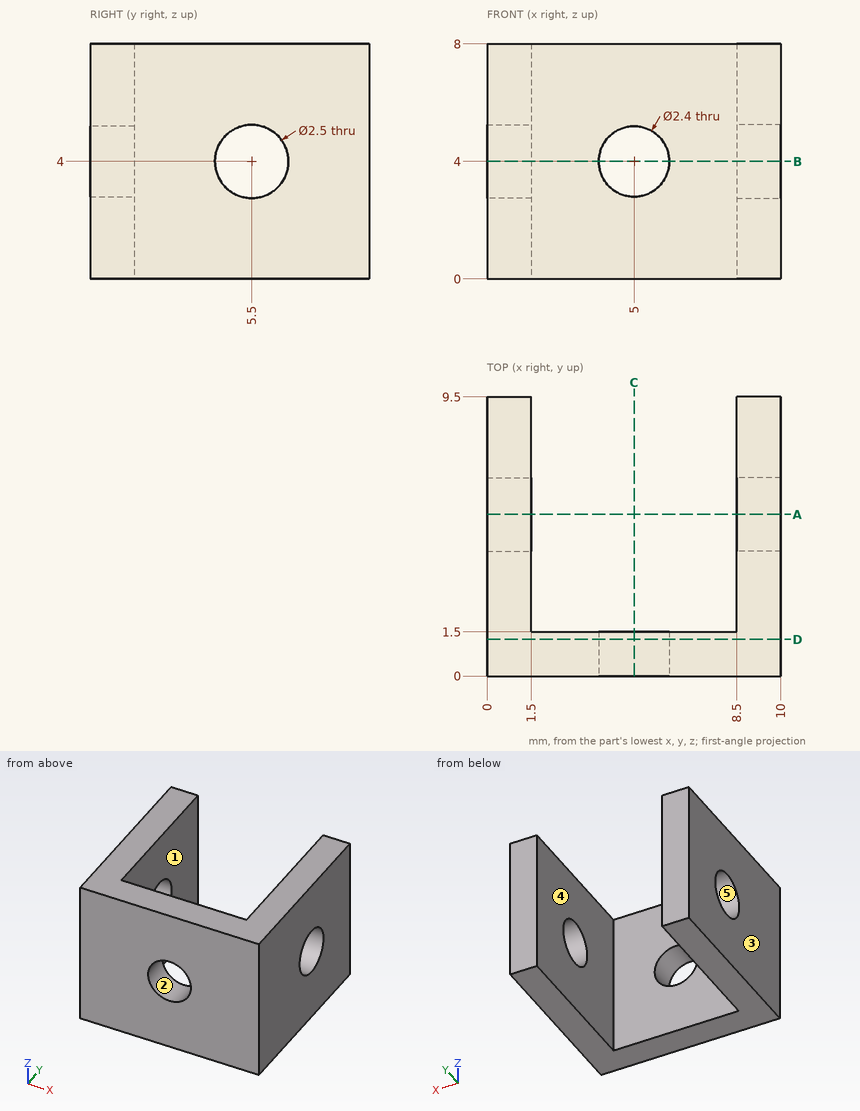
Could you check a few things on this drawing? It's one solid part, dimensions in mm from its lowest x, y, z. A direction names the side the tool comes from. Round coordinates to 2 decimals unless told otherwise and drop trailing zeros. Order: outer loops, then holes, each group sorted by start corner. A loop starts at its lowest first (then second) coordinate and runs counter-clockwise, first axis right, second up. Notation, with made-up numbers: M 85.5,-28.75 L 107.5,-28.75 A11 ccw 107.5,-10.75 Z; hole C -4,20 d6. An arc over 180 degrees is marked long. Use a Markdown table: item, result.
1) If I drill on line 1 along X through (y, z) = (7, 5); line 2 along Z through (x, y) = (5, 0.8); line 3 along X through (y, z) = (1.1, 4), over which ranges is the centre line in solid material (lowest first)?
Geometry says:
| item | result |
|---|---|
| line 1 | x = 0 to 1.5, 8.5 to 10 |
| line 2 | z = 0 to 2.8, 5.2 to 8 |
| line 3 | x = 0 to 3.8, 6.2 to 10 |
2) I'm going to push flat-ended pins straight in: P1, Ø1.5, axis at y = 5.5, z = 4, coming from the +X side; P2, Ø2, axis at x = 3.5, z = 5, coming from the +Y side. Where does each tip first touch, or does it pass through?
Geometry says:
| item | result |
|---|---|
| P1 | passes through |
| P2 | stops at y = 1.5 |
3) If we mould it in two halves opening along X, with no side actions, what happens to the marked faces 3, 4 and 5? For each: +X half, -X half, draft (parallel to the pull), parting line (faces both ways), or undercut.
Geometry says:
| item | result |
|---|---|
| face 3 | -X half |
| face 4 | undercut |
| face 5 | draft |
4) Imagine slicing it at C-C (x = 5). List the corners of the cut face in (y, z) for me.
Geometry says:
| item | result |
|---|---|
| outline | M 0,0 L 1.5,0 L 1.5,2.8 L 0,2.8 Z; M 0,5.2 L 1.5,5.2 L 1.5,8 L 0,8 Z |
5) Imagine slicing it at A-A (y = 5.5). List the corners of the cut face in (x, z) for me, then the cut area to 3 significant figures.
Geometry says:
| item | result |
|---|---|
| outline | M 0,0 L 1.5,0 L 1.5,2.75 L 0,2.75 Z; M 0,5.25 L 1.5,5.25 L 1.5,8 L 0,8 Z; M 8.5,0 L 10,0 L 10,2.75 L 8.5,2.75 Z; M 8.5,5.25 L 10,5.25 L 10,8 L 8.5,8 Z |
| area | 16.5 mm² |
6) On a 3-axis mill with a long thin cutter (end or side, diameter ignored), from which of +Z, -Z, +X, -X, +Y, -Y can I reach the whole of each face in a straight line? I mean the marked faces 1 and 2. Say none if no direction works.
Geometry says:
| item | result |
|---|---|
| face 1 | +Z, -Z, +Y |
| face 2 | +Y, -Y |
7) Imagine slicing it at B-B (z = 4). List the corners of the cut face in (x, y) for me, then the cut area to 3 significant figures.
Geometry says:
| item | result |
|---|---|
| outline | M 0,0 L 3.8,0 L 3.8,1.5 L 1.5,1.5 L 1.5,4.25 L 0,4.25 Z; M 0,6.75 L 1.5,6.75 L 1.5,9.5 L 0,9.5 Z; M 6.2,0 L 10,0 L 10,4.25 L 8.5,4.25 L 8.5,1.5 L 6.2,1.5 Z; M 8.5,6.75 L 10,6.75 L 10,9.5 L 8.5,9.5 Z |
| area | 27.9 mm² |
8) Imagine slicing it at D-D (y = 1.25). List the corners of the cut face in (x, z) for me, then the cut area to 3 significant figures.
Geometry says:
| item | result |
|---|---|
| outline | M 0,0 L 10,0 L 10,8 L 0,8 Z; hole C 5,4 d2.4 |
| area | 75.5 mm² |
